Job drawing, mm, ordinate dimensions from the low corner. One solid piece. A direction names the side the tool comes from. Round coordinates to 2 decimals unless told otherwise and drop trailing zeros. Order: outer loops, then holes, each group sorted by start corner. A loop starts at its lowest first (then second) coordinate and runs counter-clockwise, first axis right, second up. Notation, with made-up numbers: (53.5, -31) -> (58.5, -31) arc R7 cw to (58.5, -25) -> close; hole circle Ø3 at (-11.5, 21.5). An arc over 180 degrees is marked (long way). Return JSON: item names as keys, results as strings. Group by question number.
Q1. Flat gauge pins, fed straight in: pin 1 (1.1 mm diameter, centred on y = 1, z = 11, fed in from -X); pin 2 (1.8 mm diameter, centred on y = 1, z = 1.5, fed in from -X); pin 3 (1.1 mm diameter, centred on y = 2, z = 1, fed in from +X). Where does each tip first touch, or does it go through?
Q2. Cut at D-D (x = 2.25). Write the cut outline in (y, z), then the cut area to 3 significant figures.
Q3. Probe line 1 along Y through (x, z) = (4, 10.9); line 2 along X through (y, z) = (3.5, 1.4); line 3 along Y through (x, z) = (1, 7.5). List the from-to ranges inside material, lowest first.
Q4. Mould opens along X. For the marked faces 1, 2, 3 and 4 say: +X half, -X half, draft (parallel to the pull), parting line (faces both ways), or undercut.
Q5. Cut at A-A (y = 1.85). Write the cut outline in (x, z), then the cut area to 3 significant figures.
Q6. Cut at B-B (z = 6). Write the cut outline in (x, y), then the cut area to 3 significant figures.
Q7. Cut at C-C (y = 0.8). Write the cut outline in (x, z), then the cut area to 3 significant figures.
Q8. Which spindle directions (+Z, -Z, +X, -X, +Y, -Y) get a long thin tool onto all of the face, cutting with end or side? Do the marked faces 5, 6, 7, 8 and 9. Say none if no direction does.
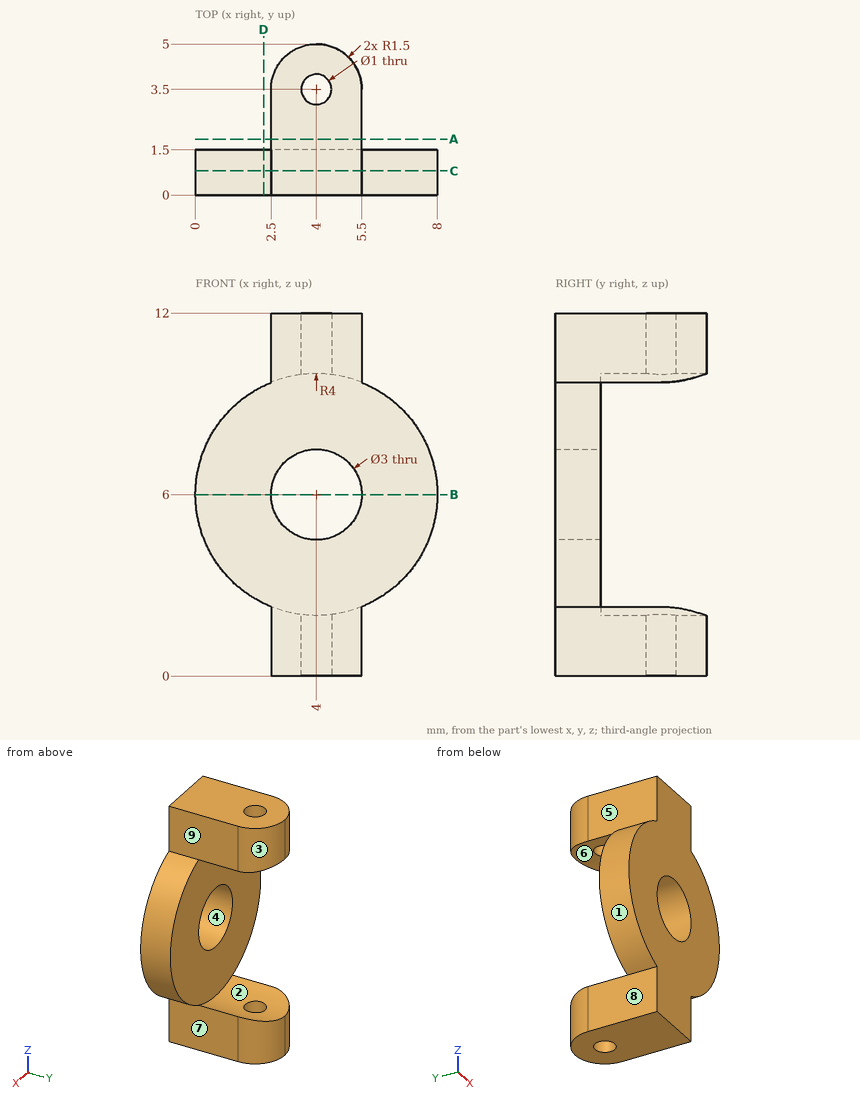
Solution:
{
 "1": {"pin 1": "stops at x = 2.5", "pin 2": "stops at x = 2.26", "pin 3": "stops at x = 5.5"},
 "2": {"outline": "(0, 2.4) -> (1.5, 2.4) -> (1.5, 9.6) -> (0, 9.6) -> close", "area": "10.8 mm²"},
 "3": {"line 1": "y = 0 to 3, 4 to 5", "line 2": "x = 2.5 to 3.5, 4.5 to 5.5", "line 3": "y = 0 to 1.5"},
 "4": {"face 1": "-X half", "face 2": "undercut", "face 3": "+X half", "face 4": "undercut"},
 "5": {"outline": "(2.5, 0) -> (5.5, 0) -> (5.5, 2.29) arc R4 cw to (2.5, 2.29) -> close; (2.5, 9.71) arc R4 cw to (5.5, 9.71) -> (5.5, 12) -> (2.5, 12) -> close", "area": "12.6 mm²"},
 "6": {"outline": "(0, 0) -> (2.5, 0) -> (2.5, 1.5) -> (0, 1.5) -> close; (5.5, 0) -> (8, 0) -> (8, 1.5) -> (5.5, 1.5) -> close", "area": "7.50 mm²"},
 "7": {"outline": "(2.5, 0) -> (5.5, 0) -> (5.5, 2.29) arc R4 ccw to (5.5, 9.71) -> (5.5, 12) -> (2.5, 12) -> (2.5, 9.71) arc R4 ccw to (2.5, 2.29) -> close; hole circle Ø3 at (4, 6)", "area": "55.8 mm²"},
 "8": {"face 5": "+Z, -X, +Y, -Y", "face 6": "+Y", "face 7": "-Z, +X, +Y, -Y", "face 8": "-Z, -X, +Y, -Y", "face 9": "+Z, +X, +Y, -Y"}
}
